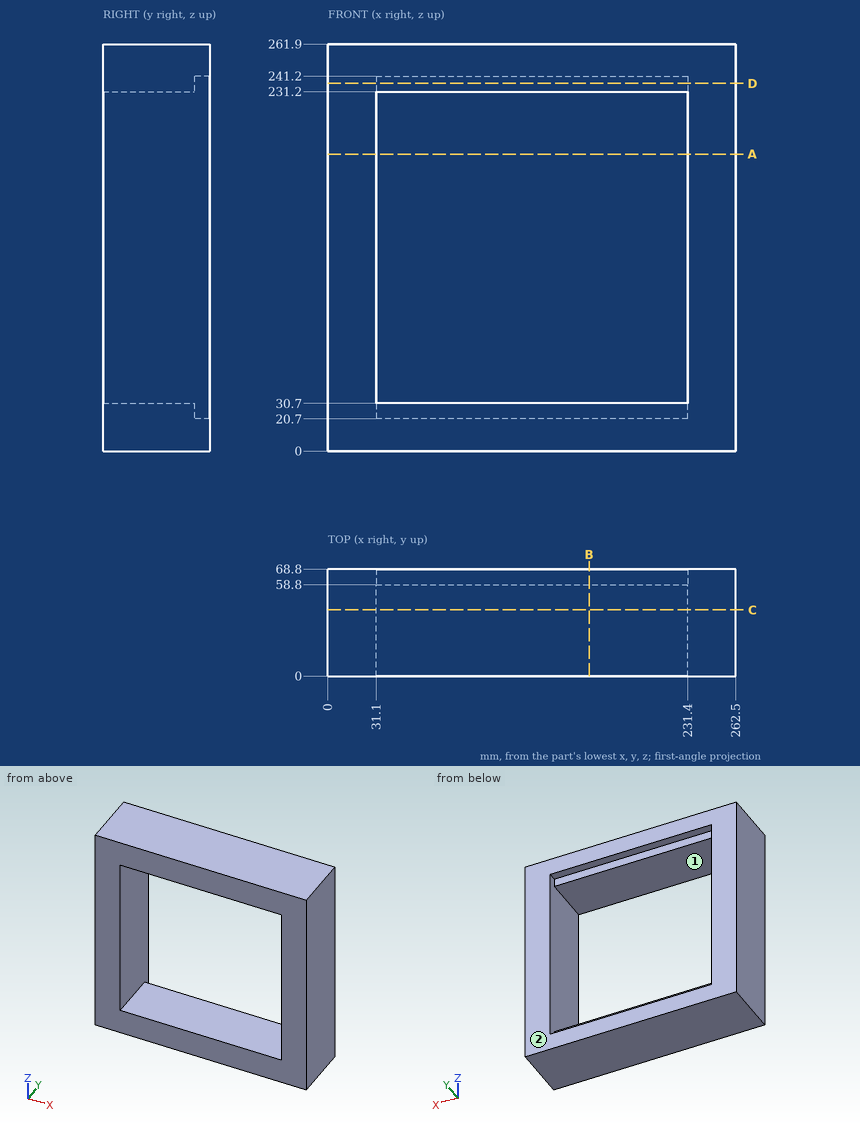
Here's the drawing with two shaded views (mm, measured from the low corner). I have some questions. A direction names the side the tool comes from. Give positions to 0.01 mm unless a question says otherwise; leave off trailing zeros. Loops run counter-clockwise (first coordinate to the right, second up) from the corner with the lowest first, then second, coordinate; pieces in that order, holes last. Notation, with made-up numbers: (14, -1.5) - (51, -1.5) arc R9 ccw to (51, 11.5) - close; hole circle Ø7 at (-15, 25). An arc over 180 degrees is marked (long way). Answer in a Markdown table with one row per item. Add a question column.
Q1. Which directions (+Z, -Z, +X, -X, +Y, -Y) give clear straight access to the entire face, cutting with the end or side of a thin tool? Please do the marked faces 1 and 2.
Q2. For pin 1 (5 mm diameter, centred on x = 141, z = 27, fed in from +Y), with a flat end and sliding along its axis, tell me the tip position at first contact or that it passes through.
Q3. If we section it at A-A (z = 191): List the corners of the cut face in (x, y) for me, plus the area to 3 significant figures.
Q4. Please list where these lines run through material, in increasing order: L1, parallel to Z at x = 131, y = 15.5; L2, parallel to X at y = 23, z = 184; L3, parallel to Z at x = 189, y = 62. Write a range as from..to.
Q5. If we section it at C-C (y = 42.5): List the corners of the cut face in (x, z) for me, plus the area to 3 significant figures.
Q6. If we section it at D-D (z = 236.5): List the corners of the cut face in (x, y) for me, plus the area to 3 significant figures.
Q7. If we section it at B-B (x = 168): List the corners of the cut face in (y, z) for me, plus the area to 3 significant figures.
The answers:
| question | item | result |
|---|---|---|
| 1 | face 1 | +Y, -Y |
| 1 | face 2 | +Z, -Z, +X, -X, +Y |
| 2 | pin 1 | stops at y = 58.8 |
| 3 | outline | (0, 0) - (31.1, 0) - (31.1, 68.8) - (0, 68.8) - close; (231.4, 0) - (262.5, 0) - (262.5, 68.8) - (231.4, 68.8) - close |
| 3 | area | 4,280 mm^2 |
| 4 | L1 | z = 0..30.7, 231.2..261.9 |
| 4 | L2 | x = 0..31.1, 231.4..262.5 |
| 4 | L3 | z = 0..20.7, 241.2..261.9 |
| 5 | outline | (0, 0) - (262.5, 0) - (262.5, 261.9) - (0, 261.9) - close; hole (31.1, 30.7) - (231.4, 30.7) - (231.4, 231.2) - (31.1, 231.2) - close |
| 5 | area | 28,600 mm^2 |
| 6 | outline | (0, 0) - (262.5, 0) - (262.5, 68.8) - (231.4, 68.8) - (231.4, 58.8) - (31.1, 58.8) - (31.1, 68.8) - (0, 68.8) - close |
| 6 | area | 16,100 mm^2 |
| 7 | outline | (0, 0) - (68.8, 0) - (68.8, 20.7) - (58.8, 20.7) - (58.8, 30.7) - (0, 30.7) - close; (0, 231.2) - (58.8, 231.2) - (58.8, 241.2) - (68.8, 241.2) - (68.8, 261.9) - (0, 261.9) - close |
| 7 | area | 4,020 mm^2 |
